from build123d import *

# Parameters (mm, degrees)
F0_R     = 200.694583
F1_DEPTH = 254
F2_T     = -2.54
F4_D     = 254


with BuildPart() as f1:
    # F0 (on Top) → F1 (new body)
    with BuildSketch(Plane.XY):
        with Locations((-5.854189, 9.84606)):
            Circle(F0_R)
    extrude(amount=F1_DEPTH)

    # F2
    f2_openings = [f1.faces().sort_by_distance(p)[0] for p in [
        (-5.854189, 9.84606, 254),
    ]]
    offset(amount=F2_T, openings=f2_openings)

    # F4 (through all)
    with Locations(Plane.XY.offset(2.54)):
        with Locations((-5.854189, 9.84606)):
            Hole(F4_D / 2)


solid = f1.part
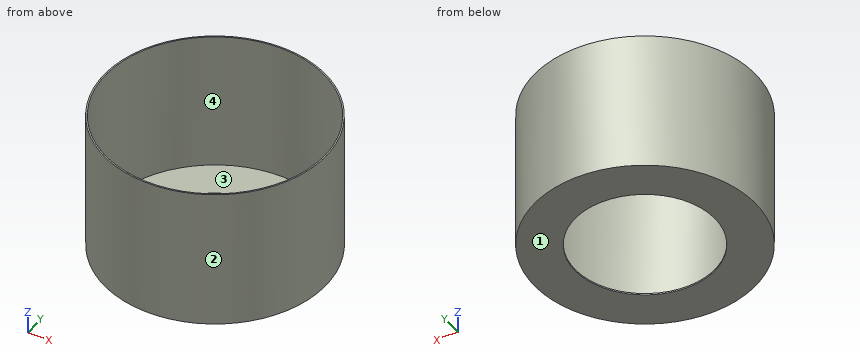
Source: CAD feature listing. Evaluate the final solid. Frame: model axes, mm. Face numbers are marked on the shaded views. Round coordinates to 2 decimals unless told otherwise and drop trailing zeros. Loops run counter-clockwise (first coordinate to the right, second up) from the corner with the lowest first, then second, coordinate; pieces in that order, holes last. Notation, with made-up numbers: M 72,35.25 L 90,35.25 A9 ccw 90,50.25 Z; hole C 82,86.25 d1. An arc over 180 degrees is marked long. Answer as CSV lines item,"result".
Q1. Cut plane C-C (x = 167.5). Return the cut outline in (y, z).
Verdict:
outline,"M -91.28,0 L 110.97,0 L 110.97,254 L 105.83,254 L 105.83,2.54 L -86.14,2.54 L -86.14,254 L -91.28,254 Z"
Q2. Cut plane A-A (y = -33.5). Return the cut outline in (x, z).
Verdict:
outline,"M -201.81,0 L -125.23,0 L -125.23,2.54 L -199.21,2.54 L -199.21,254 L -201.81,254 Z; M 113.52,0 L 190.1,0 L 190.1,254 L 187.5,254 L 187.5,2.54 L 113.52,2.54 Z"
Q3. Cut plane D-D (y = 146). Return the cut outline in (x, z), plus the area to 3 significant figures.
Verdict:
outline,"M -153.3,0 L 141.59,0 L 141.59,254 L 138.12,254 L 138.12,2.54 L -149.82,2.54 L -149.82,254 L -153.3,254 Z"
area,"2,500 mm^2"
Q4. Line query: line 1 along Z through (x, y) = (38.5, -144); line 2 along X through (y, z) = (130, 218.5); line 3 along Y through (x, z) = (29, 98). Output: solid intervals per line, ascending.
Verdict:
line 1,"z = 0 to 2.54"
line 2,"x = -166.61 to -163.42, 151.72 to 154.9"
line 3,"y = -187.8 to -185.22, 204.91 to 207.49"
Q5. Contact query for flat-ended pins moving along their axis: pin 1 (3 mm diameter, centred on y = 101, z = 132, fed in from +X); pin 2 (1.5 mm diameter, centred on x = -92, z = 211.5, fed in from -Y); pin 3 (12 mm diameter, centred on x = 83.5, z = 204, fed in from +Y). Output: stop coordinate, or through.
Verdict:
pin 1,"stops at x = 173.7"
pin 2,"stops at y = -171.77"
pin 3,"stops at y = 192.41"
Q6. Cut plane B-B (x = -68). Return the cut outline in (y, z), plus the area to 3 significant figures.
Verdict:
outline,"M -180.98,0 L -100.91,0 L -100.91,2.54 L -178.31,2.54 L -178.31,254 L -180.98,254 Z; M 120.6,0 L 200.68,0 L 200.68,254 L 198,254 L 198,2.54 L 120.6,2.54 Z"
area,"1,750 mm^2"
Q7. Pull-direction query (X, two-part tool) for the marked faces 1, 2, 3 and 4; classes: +X half, -X half, draft (parallel to the pull), parting line (faces both ways), or undercut.
Verdict:
face 1,"draft"
face 2,"parting line"
face 3,"undercut"
face 4,"undercut"
